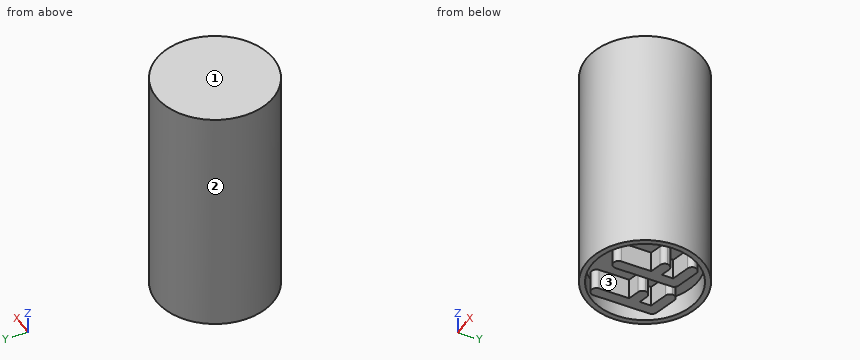
```python
from build123d import *

# Parameters (mm, degrees)
F0_R        = 5.5
F0_R_2      = 5
F1_DEPTH    = 20
F2_DEPTH    = 2
F3_R        = 0.5
F4_T1_DEPTH = 3.6258666345
F4_T3_DEPTH = 3.25
F4_T5_DEPTH = 2.959158735


# Not quite as in the source:
# - a fillet or chamfer that OpenCascade refuses, or shapes differently, is made with other operations: its cross-section is extruded or revolved along the edge and cut away or added
# - a feature names something its author has since deleted; it is built from what else it names


with BuildPart() as f1:
    # F0 (on Top) → F1 (new body)
    with BuildSketch(Plane.XY):
        with Locations((1.0606649963, 0)):
            Circle(F0_R)
        with Locations((1.0606649963, 0)):
            Circle(F0_R_2, mode=Mode.SUBTRACT)
        with Locations((1.0606649963, 0)):
            Circle(F0_R_2)
        Polygon((-1.4393350037, -3.5), (-2.4393350037, -3.5), (-2.4393350037, 2.6), (0.6516276405, 3.4282209443), (0.6516276405, 2.4282209443), (-1.4393350037, 1.8679491924), (-1.4393350037, 0.8042534147), (0.0095537358, 1.1924819824), (0.0095537358, 0.1924819824), (-1.4393350037, -0.1957465853), align=None, mode=Mode.SUBTRACT)
        Polygon((1.5606649963, -3.5), (1.5606649963, 2.6), (4.6516276405, 3.4282209443), (4.6516276405, 2.4282209443), (2.5606649963, 1.8679491924), (2.5606649963, 0.8042534147), (4.0095537358, 1.1924819824), (4.0095537358, 0.1924819824), (2.5606649963, -0.1957465853), (2.5606649963, -3.5), align=None, mode=Mode.SUBTRACT)
        Polygon((4.6516276405, 3.4282209443), (1.5606649963, 2.6), (1.5606649963, -3.5), (2.5606649963, -3.5), (2.5606649963, -0.1957465853), (4.0095537358, 0.1924819824), (4.0095537358, 1.1924819824), (2.5606649963, 0.8042534147), (2.5606649963, 1.8679491924), (4.6516276405, 2.4282209443), align=None)
        Polygon((-2.4393350037, 2.6), (-2.4393350037, -3.5), (-1.4393350037, -3.5), (-1.4393350037, -0.1957465853), (0.0095537358, 0.1924819824), (0.0095537358, 1.1924819824), (-1.4393350037, 0.8042534147), (-1.4393350037, 1.8679491924), (0.6516276405, 2.4282209443), (0.6516276405, 3.4282209443), align=None)
    extrude(amount=F1_DEPTH)

    # F0 (on Top) → F2 (join)
    with BuildSketch(Plane.XY):
        with Locations((1.0606649963, 0)):
            Circle(F0_R)
        with Locations((1.0606649963, 0)):
            Circle(F0_R_2, mode=Mode.SUBTRACT)
        Polygon((-2.4393350037, 2.6), (-2.4393350037, -3.5), (-1.4393350037, -3.5), (-1.4393350037, -0.1957465853), (0.0095537358, 0.1924819824), (0.0095537358, 1.1924819824), (-1.4393350037, 0.8042534147), (-1.4393350037, 1.8679491924), (0.6516276405, 2.4282209443), (0.6516276405, 3.4282209443), align=None)
        Polygon((4.6516276405, 3.4282209443), (1.5606649963, 2.6), (1.5606649963, -3.5), (2.5606649963, -3.5), (2.5606649963, -0.1957465853), (4.0095537358, 0.1924819824), (4.0095537358, 1.1924819824), (2.5606649963, 0.8042534147), (2.5606649963, 1.8679491924), (4.6516276405, 2.4282209443), align=None)
    extrude(amount=-F2_DEPTH)

    # F3
    f3_edges = [f1.edges().sort_by_distance(p)[0] for p in [
        (2.560665, -3.5, -1),
        (-1.439335, -3.5, -1),
        (4.009554, 0.192482, -1),
        (0.009554, 0.192482, -1),
        (4.651628, 2.428221, -1),
        (0.651628, 2.428221, -1),
    ]]
    fillet(f3_edges, radius=F3_R)

    # F4: fillet of radius 0.5 on 8 edges, made by hand

    # F4_s2 → F4_t1 (cut)
    with BuildSketch(Plane.XY.offset(-3.6258666345)):
        with BuildLine():
            ThreePointArc((4.6516276405, 2.8118844383), (4.4431733372, 3.1840141424), (4.0234410115, 3.2598988444))
            Line((4.0234410115, 3.2598988444), (4.6516276405, 3.4282209443))
            Line((4.6516276405, 3.4282209443), (4.6516276405, 2.8118844383))
        make_face()
        with BuildLine():
            ThreePointArc((0.0234410115, 3.2598988444), (0.4431733372, 3.1840141424), (0.6516276405, 2.8118844383))
            Line((0.6516276405, 2.8118844383), (0.6516276405, 3.4282209443))
            Line((0.6516276405, 3.4282209443), (0.0234410115, 3.2598988444))
        make_face()
        with BuildLine():
            ThreePointArc((0.0095537358, 0.5761454764), (-0.1989005675, 0.9482751804), (-0.6186328932, 1.0241598824))
            Line((-0.6186328932, 1.0241598824), (0.0095537358, 1.1924819824))
            Line((0.0095537358, 1.1924819824), (0.0095537358, 0.5761454764))
        make_face()
        with BuildLine():
            ThreePointArc((3.3813671068, 1.0241598824), (3.8010994325, 0.9482751804), (4.0095537358, 0.5761454764))
            Line((4.0095537358, 0.5761454764), (4.0095537358, 1.1924819824))
            Line((4.0095537358, 1.1924819824), (3.3813671068, 1.0241598824))
        make_face()
    extrude(amount=F4_T1_DEPTH, mode=Mode.SUBTRACT)

    # F4_s4 → F4_t3 (cut)
    with BuildSketch(Plane.XY.offset(-3.25)):
        with BuildLine():
            ThreePointArc((1.5606649963, -3), (1.7071116058, -3.3535533906), (2.0606649963, -3.5))
            Line((2.0606649963, -3.5), (1.5606649963, -3.5))
            Line((1.5606649963, -3.5), (1.5606649963, -3))
        make_face()
        with BuildLine():
            ThreePointArc((-1.9393350037, -3.5), (-2.2928883942, -3.3535533906), (-2.4393350037, -3))
            Line((-2.4393350037, -3), (-2.4393350037, -3.5))
            Line((-2.4393350037, -3.5), (-1.9393350037, -3.5))
        make_face()
    extrude(amount=F4_T3_DEPTH, mode=Mode.SUBTRACT)

    # F4_s6 → F4_t5 (cut)
    with BuildSketch(Plane.XY.offset(-2.959158735)):
        with BuildLine():
            ThreePointArc((1.9312554738, 2.6992994192), (1.6639883262, 2.5207172205), (1.5606649963, 2.216336506))
            Line((1.5606649963, 2.216336506), (1.5606649963, 2.6))
            Line((1.5606649963, 2.6), (1.9312554738, 2.6992994192))
        make_face()
        with BuildLine():
            ThreePointArc((-2.4393350037, 2.216336506), (-2.3360116738, 2.5207172205), (-2.0687445262, 2.6992994192))
            Line((-2.0687445262, 2.6992994192), (-2.4393350037, 2.6))
            Line((-2.4393350037, 2.6), (-2.4393350037, 2.216336506))
        make_face()
    extrude(amount=F4_T5_DEPTH, mode=Mode.SUBTRACT)


solid = f1.part
```
Geometry check sheet. Reference: the model listing, model coordinates, mm. Face numbers are marked on the shaded views. Give positions to 0.01 mm unless a question says otherwise; leave off trailing zeros. Loops run counter-clockwise (first coordinate to the right, second up) from the corner with the lowest first, then second, coordinate; pieces in that order, holes last. Notation, with made-up numbers: M 20.25,82 L 70.25,82 A16 cw 70.25,86 Z; hole C 13,42 d5. An arc over 180 degrees is marked long. Write item = value, one per line. Start each with the question number.
1. Go/stop test with flat-tipped pins: P1, Ø3, axis at y = 1.5, z = 17.5, coming from the +X side; P2, Ø1, axis at y = -1.5, z = -1, coming from the +X side; P3, Ø1.6, axis at y = -2, z = -1, coming from the +X side; P4, Ø0.6, axis at y = 0.5, z = -1, coming from the -X side. Record where each tip stops, or that it passes through.
2. Draft check along X on the marked faces 1, 2 and 3. Enter one of: +X half, -X half, draft (parallel to the pull), parting line (faces both ways), or undercut.
3. Thickness scan on probe 1 along Y at (x, z) = (2, -0.75); probe 2 along Z at (x, y) = (3.5, 3.5); probe 3 along Y at (x, z) = (0.25, 5.75). Record the ranges inside material, lowest first.
4. Section check B-B, the plane x = -3.25. Enter the section's corners in (y, z), plus the area to 3 significant figures.
5. Section check A-A, the plane y = 3.75. Enter the section's corners in (x, z).
6. Section check D-D, the plane y = -2. Enter the section's corners in (x, z).
7. Section check C-C, the plane z = 8.25. Enter the section's corners in (x, y).
Values follow:
q1.P1 = 6.56
q1.P2 = 6.47
q1.P3 = 6.43
q1.P4 = -4.44
q2.face_1 = draft
q2.face_2 = parting line
q2.face_3 = undercut
q3.probe_1 = -5.42 to -4.91, -3.5 to 2.72, 4.91 to 5.42
q3.probe_2 = 0 to 20
q3.probe_3 = -5.44 to 5.44
q4.outline = M -3.42,-2 L -2.53,-2 L -2.53,0 L 2.53,0 L 2.53,-2 L 3.42,-2 L 3.42,20 L -3.42,20 Z
q4.area = 140 mm^2
q5.outline = M -2.96,-2 L -2.25,-2 L -2.25,0 L 4.37,0 L 4.37,-2 L 5.08,-2 L 5.08,20 L -2.96,20 Z
q6.outline = M -4.06,-2 L -3.52,-2 L -3.52,0 L -2.44,0 L -2.44,-2 L -1.44,-2 L -1.44,0 L 1.56,0 L 1.56,-2 L 2.56,-2 L 2.56,0 L 5.64,0 L 5.64,-2 L 6.18,-2 L 6.18,20 L -4.06,20 Z
q7.outline = C 1.06,0 d11
